Part model, mm, in its own coordinate system. A direction names the side the tool comes from. Give positions to 0.01 mm unless a question says otherwise; leave off trailing zeros. Write each loop counter-clockwise with the first axis right and the second up, starting at its lowest first coordinate (ties: lowest second). Pieces come first, ordered by that corner, then holes. Notation, with made-up numbers: M 32,64 L 87,64 A22 ccw 87,82 Z; hole C 21,34.5 d9. An arc over 180 degrees is marked long. Use CSV: the item, a comma, the result in double quotes. Start each with the question number.
Item 1: Mould opens along X. For faces 1 (the flat face through (21, -1.5, 12)), 2 (the flat face through (22, 0, 12)), 3 (the flat face through (-19, 0, 24)) say: released by +X, released by -X, zero draft, split by the parting line, or undercut.
Item 2: Which spindle directions (+Z, -Z, +X, -X, +Y, -Y) get a long thin tool onto all of the face, cutting with end or side? Do faces 4 (the flat face through (18, 4, 13)), 5 (the cylindrical face through (12.295, 12.454, 12.325)), 6 (the flat face through (-21, 1.5, 12)), 7 (the flat face through (-18, 2, 2.5)). Say none if no direction does.
Item 3: Cut at B-B (y = 2.5). List the corners of the cut face in (x, z).
Item 4: Drill centre lines: line 1 (X direction, y = 1, z = 21.25); line 2 (Y direction, x = 4, z = 17.75); line 3 (Y direction, x = -1.5, z = 2.25). Where is each one in solid material? Low to high. Write a range as [from, to].
Item 5: Cut at C-C (y = 11.75). List the corners of the cut face in (x, z), then the cut area to 3 significant figures.
Item 6: Cut at A-A (z = 15.5). List the corners of the cut face in (x, y), then the cut area to 3 significant figures.
Item 7: Pin check, flat tips, straight feed: pin 1 (1.7 mm diameter, centred on x = 17.5, z = 9.5, fed in from -Y); pin 2 (5 mm diameter, centred on x = 5, z = 13, fed in from +Y); pin 3 (5 mm diameter, centred on y = 11.5, z = 3, fed in from -X). Stop position of each tip, or through.
Item 8: Cut at D-D (x = -18). List the corners of the cut face in (y, z), then the cut area to 3 significant figures.
from build123d import *

# Parameters (mm, degrees)
F1_DEPTH = 25
F3_DEPTH = 25
F4_W     = 41
F4_H     = 20
F5_DEPTH = 4


with BuildPart() as f1:
    # F0 (on Top) → F1 (new body)
    with BuildSketch(Plane.XY):
        with BuildLine():
            ThreePointArc((-17.5, 0), (0, 17.5), (17.5, 0))
            Line((17.5, 0), (20.5, 0))
            Line((20.5, 0), (20.5, -1.5))
            Line((20.5, -1.5), (22, -1.5))
            Line((22, -1.5), (22, 1.5))
            Line((22, 1.5), (18.940697, 1.5))
            ThreePointArc((18.940697, 1.5), (0, 19), (-18.940697, 1.5))
            Line((-18.940697, 1.5), (-22, 1.5))
            Line((-22, 1.5), (-22, -1.5))
            Line((-22, -1.5), (-20.5, -1.5))
            Line((-20.5, -1.5), (-20.5, 0))
            Line((-20.5, 0), (-17.5, 0))
        make_face()
    extrude(amount=F1_DEPTH)

    # F2 (on face) → F3 (join)
    with BuildSketch(Plane.XY.offset(25)):
        with BuildLine():
            Line((5, 16.77051), (5, 18.330303))
            ThreePointArc((5, 18.330303), (0, 19), (-5, 18.330303))
            Line((-5, 18.330303), (-5, 16.77051))
            Line((-5, 16.77051), (5, 16.77051))
        make_face()
    extrude(amount=-F3_DEPTH)

    # F4 (on face) → F5 (cut)
    with BuildSketch(Plane.XZ):
        with Locations((0, 12.5)):
            Rectangle(F4_W, F4_H)
    extrude(amount=-F5_DEPTH, mode=Mode.SUBTRACT)


solid = f1.part
Worked answers:
1,face 1,"zero draft"
1,face 2,"released by +X"
1,face 3,"undercut"
2,face 4,"+X, -X, -Y"
2,face 5,"+Z, -Z, -Y"
2,face 6,"+Z, -Z, -X, +Y"
2,face 7,"-Y"
3,outline,"M -18.83,0 L -17.32,0 L -17.32,2.5 L -18.83,2.5 Z; M -18.83,22.5 L -17.32,22.5 L -17.32,25 L -18.83,25 Z; M 17.32,0 L 18.83,0 L 18.83,2.5 L 17.32,2.5 Z; M 17.32,22.5 L 18.83,22.5 L 18.83,25 L 17.32,25 Z"
4,line 1,"x = [-22, -20.5], [20.5, 22]"
4,line 2,"y = [16.77, 18.57]"
4,line 3,"y = [16.77, 18.94]"
5,outline,"M -14.93,0 L -12.97,0 L -12.97,25 L -14.93,25 Z; M 12.97,0 L 14.93,0 L 14.93,25 L 12.97,25 Z"
5,area,"98.1 mm^2"
6,outline,"M -22,-1.5 L -20.5,-1.5 L -20.5,1.5 L -22,1.5 Z; M -18.57,4 L -17.04,4 A17.5 cw -5,16.77 L 5,16.77 A17.5 cw 17.04,4 L 18.57,4 A19 ccw 5,18.33 A19 ccw -5,18.33 A19 ccw Z; M 20.5,-1.5 L 22,-1.5 L 22,1.5 L 20.5,1.5 Z"
6,area,"87.8 mm^2"
7,pin 1,"stops at y = 4"
7,pin 2,"stops at y = 18.83"
7,pin 3,"stops at x = -16.73"
8,outline,"M 0,0 L 6.08,0 L 6.08,25 L 0,25 L 0,22.5 L 4,22.5 L 4,2.5 L 0,2.5 Z"
8,area,"72.1 mm^2"
